Read the model definition and answer for the solid it produces. Units are mm, in the model's axes. A direction names the side the tool comes from. Coordinates: 2 decimals unless noted, no trailing zeros. Loops run counter-clockwise (first coordinate to the right, second up) from the corner with the lowest first, then second, coordinate; pieces in that order, holes last. Notation, with made-up numbers: (35.5, 36) -> (89.5, 36) arc R22 ccw to (89.5, 73) -> close; hole circle Ø4 at (18.25, 66). An arc over 180 degrees is marked (long way). Answer as a JSON object with one key per item and string values. Group by question number.
1) Which of the six approach directions +Z, -Z, +X, -X, +Y, -Y give full straight-line access (tool end or side, diameter ignored) to faces 4 (the face through (-29.955, 49.875, 1.479)), 5 (the face through (-44.47, 45.54, 1.48)), 6 (the face through (-31.827, 21.504, 1.479))?
2) Section B-B, the plane z = 1.05 is taken. Give the vertices of the cut face in (x, y) (3 decimals), plus the area to 3 significant figures.
3) Section D-D, the plane y = 24 is taken. Give the vertices of the cut face in (x, z).
4) Determine the mould class of faces 1 (the face through (-31.083, 46.334, 1.479)), 2 (the face through (-27, 35, 3)), 3 (the face through (-37.503, 33.025, 1.479)) for opening direction X: released by +X, released by -X, zero draft, split by the parting line, or undercut.
5) Consider probe 1 along Y at (x, z) = (-33, 1.25); probe 2 along X at (y, z) = (45.5, 0.1); probe 3 along Y at (x, z) = (-37, 0.6). Determine where each line is inside the solid, lowest interval first. Write a range as [from, to].
6) Section C-C, the plane x = -33.5 is taken. Give the vertices of the cut face in (y, z).
7) Flat-ended cylindrical pins translate along their axes: P1, Ø2.5, axis at x = -40.31, y = 40.31, coming from the -Z side; P2, Ø1.5, axis at x = -39.5, z = 1.5, coming from the +Y side; P3, Ø1, axis at y = 42.5, z = 2, coming from the -X side. Find the tip coordinate at first contact, or state that the pin passes through.
8) Section A-A, the plane y = 47 is taken. Give the vertices of the cut face in (x, z), plus the area to 3 significant figures.
from build123d import *

# Parameters (mm, degrees)
BOSS_EXTRUDE1_DEPTH     = 115
BOSS_EXTRUDE2_DEPTH     = 3
SKETCH4_R               = 1.65
CUT_EXTRUDE1_DEPTH      = 116
CUT_EXTRUDE2_DEPTH      = 116
CUT_EXTRUDE_THIN1_DEPTH = 116
CUT_EXTRUDE3_DEPTH      = 116


with BuildPart() as part:
    # Sketch1 → Boss-Extrude1 (new body)
    with BuildSketch(Plane(origin=(0, 0, 0), x_dir=(0, 1, 0), z_dir=(0, 0, 1))):
        with BuildLine():
            Line((66.793011614, 25.63943495), (62.125109481, 23.847595202))
            ThreePointArc((62.125109481, 23.847595202), (50.18784505, 43.696878999), (32.170193606, 58.252173078))
            Line((32.170193606, 58.252173078), (34.587369472, 62.629073903))
            ThreePointArc((34.587369472, 62.629073903), (53.95881545, 46.980136869), (66.793011614, 25.63943495))
        make_face()
    extrude(amount=BOSS_EXTRUDE1_DEPTH)

    # Sketch3 → Boss-Extrude2 (add)
    with BuildSketch(Plane(origin=(0, 0, 0), x_dir=(0, 1, 0), z_dir=(0, 0, 1))):
        with BuildLine():
            ThreePointArc((37.772226983, 9.055581263), (42.402339681, 14.205235152), (43.997873295, 20.944014808))
            ThreePointArc((43.997873295, 20.944014808), (49.930251766, 28.811968202), (58.997685125, 24.954578252))
            ThreePointArc((58.997685125, 24.954578252), (60.351321071, 23.807583941), (62.125109481, 23.847595202))
            ThreePointArc((62.125109481, 23.847595202), (50.18784505, 43.696878999), (32.170193606, 58.252173078))
            ThreePointArc((32.170193606, 58.252173078), (31.867825608, 56.602303211), (32.676329677, 55.132671232))
            ThreePointArc((32.676329677, 55.132671232), (36.307290349, 43.066223982), (27.152640183, 34.407390053))
            ThreePointArc((27.152640183, 34.407390053), (21.43315886, 31.77290535), (17.44684462, 26.898248947))
            ThreePointArc((17.44684462, 26.898248947), (17.417631935, 26.825058047), (17.400281887, 26.748186307))
            ThreePointArc((17.400281887, 26.748186307), (22.701893313, 12.386399614), (37.629460858, 8.989970916))
            ThreePointArc((37.629460858, 8.989970916), (37.70343721, 9.017133171), (37.772226983, 9.055581263))
        make_face()
    extrude(amount=BOSS_EXTRUDE2_DEPTH)

    # Sketch4 → Cut-Extrude1 (cut, through all)
    with BuildSketch(Plane(origin=(0, 0, 0), x_dir=(0, 1, 0), z_dir=(0, 0, 1))):
        with Locations((40.305086528, 40.305086528)):
            Circle(SKETCH4_R)
        with Locations((46.691666524, 32.693856872)):
            Circle(SKETCH4_R)
    extrude(amount=CUT_EXTRUDE1_DEPTH, mode=Mode.SUBTRACT)

    # Sketch6 → Cut-Extrude2 (cut, through all)
    with BuildSketch(Plane(origin=(0, 0, 0), x_dir=(0, 1, 0), z_dir=(0, 0, 1))):
        with BuildLine():
            ThreePointArc((52.744660964, 40.57385568), (56.433360559, 35.263477438), (59.589277435, 29.620179604))
            Line((59.589277435, 29.620179604), (53.604790209, 29.411196706))
            ThreePointArc((53.604790209, 29.411196706), (50.072999838, 31.289082957), (49.933401851, 35.286646265))
            Line((49.933401851, 35.286646265), (52.744660964, 40.57385568))
        make_face()
        with BuildLine():
            ThreePointArc((38.577322779, 54.222017596), (43.657448084, 50.222149016), (48.32540701, 45.748137255))
            Line((48.32540701, 45.748137255), (42.663514101, 43.798591183))
            ThreePointArc((42.663514101, 43.798591183), (38.737005367, 44.561827164), (37.434732749, 48.343901467))
            Line((37.434732749, 48.343901467), (38.577322779, 54.222017596))
        make_face()
    extrude(amount=CUT_EXTRUDE2_DEPTH, mode=Mode.SUBTRACT)

    # Sketch6_4 → Cut-Extrude-Thin1 (cut, through all)
    with BuildSketch(Plane(origin=(0, 0, 0), x_dir=(0, 1, 0), z_dir=(0, 0, 1))):
        with BuildLine():
            Line((60.063470687, 29.336555934), (53.615260058, 29.111379457))
            ThreePointArc((53.615260058, 29.111379457), (49.818585409, 31.130107177), (49.668517573, 35.427487734))
            Line((49.668517573, 35.427487734), (52.697614338, 41.124390185))
            ThreePointArc((52.697614338, 41.124390185), (56.687774988, 35.422453218), (60.063470687, 29.336555934))
        make_face()
        with BuildLine():
            Line((59.589277435, 29.620179604), (53.604790209, 29.411196706))
            ThreePointArc((53.604790209, 29.411196706), (50.072999838, 31.289082957), (49.933401851, 35.286646265))
            Line((49.933401851, 35.286646265), (52.744660964, 40.57385568))
            ThreePointArc((52.744660964, 40.57385568), (56.433360559, 35.263477438), (59.589277435, 29.620179604))
        make_face(mode=Mode.SUBTRACT)
        with BuildLine():
            Line((48.861803808, 45.61554728), (42.761184547, 43.51493561))
            ThreePointArc((42.761184547, 43.51493561), (38.540187658, 44.33541429), (37.140244594, 48.401144165))
            Line((37.140244594, 48.401144165), (38.371371155, 54.734741259))
            ThreePointArc((38.371371155, 54.734741259), (43.854265793, 50.44856189), (48.861803808, 45.61554728))
        make_face()
        with BuildLine():
            Line((48.32540701, 45.748137255), (42.663514101, 43.798591183))
            ThreePointArc((42.663514101, 43.798591183), (38.737005367, 44.561827164), (37.434732749, 48.343901467))
            Line((37.434732749, 48.343901467), (38.577322779, 54.222017596))
            ThreePointArc((38.577322779, 54.222017596), (43.657448084, 50.222149016), (48.32540701, 45.748137255))
        make_face(mode=Mode.SUBTRACT)
    extrude(amount=CUT_EXTRUDE_THIN1_DEPTH, mode=Mode.SUBTRACT)

    # Sketch7 → Cut-Extrude3 (cut, through all)
    with BuildSketch(Plane(origin=(0, 0, 0), x_dir=(0, 1, 0), z_dir=(0, 0, 1))):
        with BuildLine():
            Line((48.240089186, 45.401473768), (38.540187658, 44.33541429))
            Line((38.540187658, 44.33541429), (36.307290349, 43.066223982))
            Line((36.307290349, 43.066223982), (22.600693744, 60.972682424))
            Line((22.600693744, 60.972682424), (52.388918832, 72.501111316))
            Line((52.388918832, 72.501111316), (73.007988399, 34.26459203))
            Line((73.007988399, 34.26459203), (68.951063276, 18.611622597))
            Line((68.951063276, 18.611622597), (52.388918832, 26.438107314))
            Line((52.388918832, 26.438107314), (49.930251766, 28.811968202))
            Line((49.930251766, 28.811968202), (49.818585409, 31.130107177))
            Line((49.818585409, 31.130107177), (52.388918832, 40.543818378))
            ThreePointArc((52.388918832, 40.543818378), (50.373093191, 43.022685962), (48.240089186, 45.401473768))
        make_face()
    extrude(amount=CUT_EXTRUDE3_DEPTH, mode=Mode.SUBTRACT)


solid = part.part
Determined:
{
 "1": {"face 4": "+Z, -Z, +Y", "face 5": "+Z, -Z, -X", "face 6": "+Z, -Z, -X, -Y"},
 "2": {"outline": "(-45.401, 48.24) -> (-43.515, 42.761) arc R4.3 cw to (-44.335, 38.54) -> (-43.066, 36.307) arc R12 cw to (-34.407, 27.153) arc R14 ccw to (-26.898, 17.447) arc R0.5 ccw to (-26.748, 17.4) arc R16.062 ccw to (-8.99, 37.629) arc R0.5 ccw to (-9.056, 37.772) arc R14 ccw to (-20.944, 43.998) arc R8 cw to (-28.812, 49.93) -> (-31.13, 49.819) arc R4.3 cw to (-35.427, 49.669) -> (-40.544, 52.389) arc R66.245 ccw to start; hole circle Ø3.3 at (-40.305, 40.305); hole circle Ø3.3 at (-32.694, 46.692)", "area": "778 mm²"},
 "3": {"outline": "(-33.35, 0) -> (-11.36, 0) -> (-11.36, 3) -> (-33.35, 3) -> close"},
 "4": {"face 1": "undercut", "face 2": "zero draft", "face 3": "released by -X"},
 "5": {"probe 1": "[23.31, 45.07], [48.31, 49.18]", "probe 2": "[-44.46, -33.84], [-31.55, -25.75]", "probe 3": "[32.47, 50.5]"},
 "6": {"outline": "(24.33, 0) -> (45.25, 0) -> (45.25, 3) -> (24.33, 3) -> close; (48.13, 0) -> (49.17, 0) -> (49.17, 3) -> (48.13, 3) -> close"},
 "7": {"P1": "through", "P2": "y = 52.23", "P3": "x = -43.6"},
 "8": {"outline": "(-44.97, 0) -> (-34.31, 0) -> (-34.31, 3) -> (-44.97, 3) -> close; (-31.07, 0) -> (-27.33, 0) -> (-27.33, 3) -> (-31.07, 3) -> close", "area": "43.2 mm²"}
}
